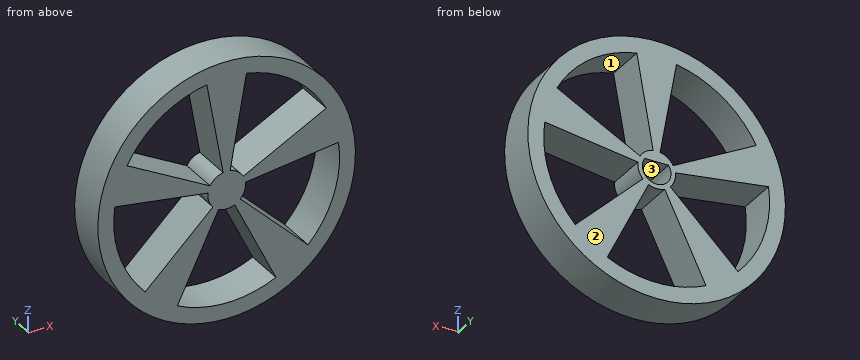
from build123d import *

# Parameters (mm, degrees)
SKETCH1_R           = 12.153059969
BOSS_EXTRUDE1_DEPTH = 3.81
SKETCH1_8_R         = 1.350728719
BOSS_EXTRUDE3_DEPTH = 0.254


with BuildPart() as part:
    # Sketch1 → Boss-Extrude1 (new body)
    with BuildSketch(Plane(origin=(0, 0, 0), x_dir=(1, 0, 0), z_dir=(0, 1, 0))):
        with Locations(Location((0, 0, 0), (0, 0, 90))):
            Circle(SKETCH1_R)
        with BuildLine():
            Line((1.870310758, -10.493185668), (0.32820092, -1.747446181))
            ThreePointArc((0.32820092, -1.747446181), (1.045082179, -1.438432216), (1.560500416, -0.85212819))
            Line((1.560500416, -0.85212819), (9.401654798, -5.02134393))
            ThreePointArc((9.401654798, -5.02134393), (6.264947316, -8.622960218), (1.870310758, -10.493185668))
        make_face(mode=Mode.SUBTRACT)
        with BuildLine():
            Line((10.557570415, -1.463801463), (1.763339739, -0.227852943))
            ThreePointArc((1.763339739, -0.227852943), (1.690978486, 0.549432216), (1.292643216, 1.220801997))
            Line((1.292643216, 1.220801997), (7.680852973, 7.38982445))
            ThreePointArc((7.680852973, 7.38982445), (10.136897695, 3.29367772), (10.557570415, -1.463801463))
        make_face(mode=Mode.SUBTRACT)
        with BuildLine():
            Line((4.654626598, 9.588506611), (0.761602973, 1.606625318))
            ThreePointArc((0.761602973, 1.606625318), (0, 1.778), (-0.761602973, 1.606625318))
            Line((-0.761602973, 1.606625318), (-4.654626598, 9.588506611))
            ThreePointArc((-4.654626598, 9.588506611), (0, 10.658564997), (4.654626598, 9.588506611))
        make_face(mode=Mode.SUBTRACT)
        with BuildLine():
            Line((-7.680852973, 7.38982445), (-1.292643216, 1.220801997))
            ThreePointArc((-1.292643216, 1.220801997), (-1.690978486, 0.549432216), (-1.763339739, -0.227852943))
            Line((-1.763339739, -0.227852943), (-10.557570415, -1.463801463))
            ThreePointArc((-10.557570415, -1.463801463), (-10.136897695, 3.29367772), (-7.680852973, 7.38982445))
        make_face(mode=Mode.SUBTRACT)
        with BuildLine():
            Line((-9.401654798, -5.02134393), (-1.560500416, -0.85212819))
            ThreePointArc((-1.560500416, -0.85212819), (-1.045082179, -1.438432216), (-0.32820092, -1.747446181))
            Line((-0.32820092, -1.747446181), (-1.870310758, -10.493185668))
            ThreePointArc((-1.870310758, -10.493185668), (-6.264947316, -8.622960218), (-9.401654798, -5.02134393))
        make_face(mode=Mode.SUBTRACT)
        with BuildLine():
            Line((1.11526861, -0.762), (-1.11526861, -0.762))
            ThreePointArc((-1.11526861, -0.762), (0, 1.350728719), (1.11526861, -0.762))
        make_face(mode=Mode.SUBTRACT)
    extrude(amount=BOSS_EXTRUDE1_DEPTH)

    # Sketch1_8 → Boss-Extrude3 (add)
    with BuildSketch(Plane(origin=(0, 0, 0), x_dir=(1, 0, 0), z_dir=(0, 1, 0))):
        Circle(SKETCH1_8_R)
    extrude(amount=BOSS_EXTRUDE3_DEPTH)


solid = part.part
Geometry check sheet. Reference: the model listing, model coordinates, mm. Face numbers are marked on the shaded views. A direction names the side the tool comes from. Give positions to 0.01 mm unless a question says otherwise; leave off trailing zeros. Loops run counter-clockwise (first coordinate to the right, second up) from the corner with the lowest first, then second, coordinate; pieces in that order, holes last. Notation, with made-up numbers: M -27,69.25 L 12,69.25 A22 cw 12,87.25 Z; hole C 22.25,67 d8. An arc over 180 degrees is marked long. Write each question's results on one line, items separated by ' | '.
1) Thickness scan on line 1 (X direction, y = 2.3, z = 0); line 2 (X direction, y = 3.15, z = 3); line 3 (Z direction, x = -4.75, y = 3.55). Record the ranges inside material, lowest first.
Answers follow:
line 1: -12.15 to -10.66, -1.78 to -1.35, 1.35 to 1.78, 10.66 to 12.15 | line 2: -11.78 to -5.6, -0.55 to 0.55, 5.6 to 11.78 | line 3: -11.19 to -4.56, 0.65 to 2.55, 9.54 to 11.19
2) Section check A-A, the plane x = 0. Record the boundary of the cut face in (y, z), plus the area to 3 significant figures.
Answers follow:
outline: M 0,-12.15 L 3.81,-12.15 L 3.81,-10.66 L 0,-10.66 Z; M 0,-1.78 L 3.81,-1.78 L 3.81,-1.35 L 0.25,-1.35 L 0.25,0.76 L 3.81,0.76 L 3.81,12.15 L 0,12.15 Z | area: 51.3 mm2
3) Gauge pin test, flat ends, axial feed: pin 1 (2 mm diameter, centred on x = -9.5, y = 2.5, fed in from -Z); pin 2 (1.5 mm diameter, centred on x = 8.5, y = 2.5, fed in from -Z); pin 3 (1 mm diameter, centred on x = -7, z = -4.5, fed in from -Y); pin 4 (2 mm diameter, centred on x = -2, y = 3, fed in from +Z). Record the tip position at first contact, or that the pin passes through.
Answers follow:
pin 1: z = -8.69 | pin 2: z = -9.36 | pin 3: through | pin 4: z = 12.11
4) Tool access check on the marked faces 1, 2 and 3. Record the directions out of +Z, -Z, +X, -X, +Y, -Y that give a thin tool (end or side, any length) a straight path to the whole face; none if there is none.
Answers follow:
face 1: +Y, -Y | face 2: +Z, -Z, +X, -X, +Y | face 3: +Y
5) Section check C-C, the plane y = 2.75. Record the boundary of the cut face in (x, z), plus the area to 3 significant figures.
Answers follow:
outline: C 0,0 d24.31; hole M -10.56,1.46 A10.66 ccw -7.68,-7.39 L -1.29,-1.22 A1.78 cw -1.76,0.23 Z; hole M -9.4,5.02 L -1.56,0.85 A1.78 cw -0.33,1.75 L -1.87,10.49 A10.66 ccw Z; hole M -4.65,-9.59 A10.66 ccw 4.65,-9.59 L 0.76,-1.61 A1.78 cw -0.76,-1.61 Z; hole M -1.12,0.76 A1.35 ccw long 1.12,0.76 Z; hole M 0.33,1.75 A1.78 cw 1.56,0.85 L 9.4,5.02 A10.66 ccw 1.87,10.49 Z; hole M 1.29,-1.22 L 7.68,-7.39 A10.66 ccw 10.56,1.46 L 1.76,0.23 A1.78 cw Z | area: 210 mm2
6) Section check B-B, the plane z = 4.25. Record the boundary of the cut face in (x, y).
Answers follow:
outline: M -11.39,0 L -7.95,0 L -7.95,3.81 L -11.39,3.81 Z; M -0.77,0 L 0.77,0 L 0.77,3.81 L -0.77,3.81 Z; M 7.95,0 L 11.39,0 L 11.39,3.81 L 7.95,3.81 Z
7) Section check D-D, the plane x = -3.5. Record the boundary of the cut face in (y, z).
Answers follow:
outline: M 0,-11.64 L 3.81,-11.64 L 3.81,-10.07 L 0,-10.07 Z; M 0,-7.22 L 3.81,-7.22 L 3.81,-3.35 L 0,-3.35 Z; M 0,0.47 L 3.81,0.47 L 3.81,1.88 L 0,1.88 Z; M 0,10.07 L 3.81,10.07 L 3.81,11.64 L 0,11.64 Z
